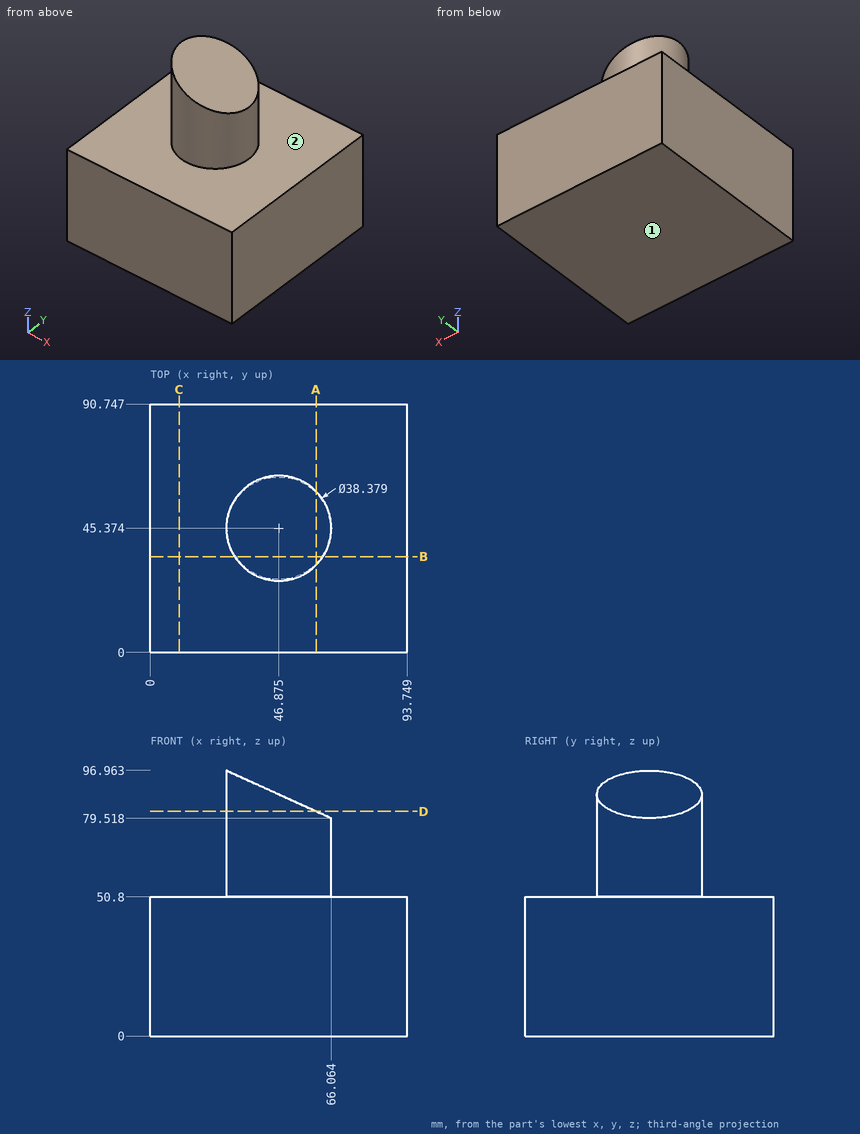
For this review, use the dimensioned drawing (mm, ordinates from the lowest corner) and the shaded views. A direction names the side the tool comes from. Coordinates: 2 decimals unless noted, no trailing zeros. Write each loop counter-clockwise with the first axis right and the second up, starting at its lowest first coordinate (ties: lowest second). Pieces come first, ordered by that corner, then holes. Notation, with made-up numbers: (15, -38) - (58, -38) arc R19 ccw to (58, -24) - close; hole circle Ø6 at (84.25, 17). An arc over 180 degrees is marked (long way). Answer as a JSON object with one key per item and string values. Group by question number.
1. Clearance check with flat-ended pins moving along their axes: pin 1 Ø8 at (x, z) = (50.5, 85.5) entering from +Y; pin 2 Ø3 at (x, y) = (11.5, 32.5) entering from +Z; pin 3 Ø8 at (y, z) = (72.5, 61) entering from -X; pin 4 Ø6 at (y, z) = (37, 57) entering from -X. State where each tip first meets the part, or that it passes through.
2. Machinability: for the marked faces 1 and 2, which of the approach directions +Z, -Z, +X, -X, +Y, -Y give a long, thin tool a straight path to every point of the face, cutting with its end or side? Answer none if there is none.
3. Add section D-D (z = 82). Give the boundary of the cut face in (x, y) (1 decimal).
4. Add section A-A (x = 60.5). Give the boundary of the cut face in (y, z) (1 decimal).
5. Add section C-C (x = 10.5). Give the boundary of the cut face in (y, z).
6. To check wall thickness, follow probe 1 along Z at (x, y) = (67, 10); probe 2 along X at (y, z) = (52.5, 54); probe 3 along X at (y, z) = (34, 53). State the ranges of each line that lie inside material, in increasing order.
7. Add section B-B (y = 35). Give the boundary of the cut face in (x, z), plus the area to 3 significant figures.
Findings:
{
 "1": {"pin 1": "y = 64.56", "pin 2": "z = 50.8", "pin 3": "through", "pin 4": "x = 28.45"},
 "2": {"face 1": "-Z, +X, -X, +Y, -Y", "face 2": "+Z"},
 "3": {"outline": "(60.6, 32) - (60.6, 58.8) arc R19.2 ccw (long way) to start"},
 "4": {"outline": "(0, 0) - (90.7, 0) - (90.7, 50.8) - (58.9, 50.8) - (58.9, 82) - (31.9, 82) - (31.9, 50.8) - (0, 50.8) - close"},
 "5": {"outline": "(0, 0) - (90.75, 0) - (90.75, 50.8) - (0, 50.8) - close"},
 "6": {"probe 1": "0 to 50.8", "probe 2": "29.06 to 64.69", "probe 3": "31.42 to 62.33"},
 "7": {"outline": "(0, 0) - (93.75, 0) - (93.75, 50.8) - (63.02, 50.8) - (63.02, 80.9) - (30.73, 95.58) - (30.73, 50.8) - (0, 50.8) - close", "area": "5,970 mm²"}
}
